CAD build for the part. Positions are in the model's coordinates, mm. Give positions to 0.01 mm unless a question says otherwise; leave off trailing zeros. Loops run counter-clockwise (first coordinate to the right, second up) from the corner with the lowest first, then second, coordinate; pieces in that order, holes last. Notation, with made-up numbers: M 47,89 L 56,89 A14 ccw 56,103 Z; hole C 73.5,36 d3. An arc over 180 degrees is marked long. Answer as CSV lines item,"result".
```python
from build123d import *

# Parameters (mm, degrees)
SKETCH_1_R       = 4.175
EXTRUDE_1_DEPTH  = 5
FILLET_1_DEPTH   = 5
FILLET_1_2_DEPTH = 5


with BuildPart() as part:
    # ｽｹｯﾁ1 → ﾎﾞｽ - 押し出し1 (new body)
    # profile 1 of 4: a face of its own
    with BuildSketch(Plane(origin=(0, 0, 0), x_dir=(1, 0, 0), z_dir=(0, 1, 0))):
        Polygon((21.537147831, 13.436802865), (14.676517829, 20.712224225), (-21.537147831, -13.436802865), (-14.676517829, -20.712224225), align=None)
        with Locations(Location((-12.65026681, -11.929041043, 0), (0, 0, 270))):
            Circle(SKETCH_1_R, mode=Mode.SUBTRACT)
        with Locations(Location((5.538286591, 5.222533963, 0), (0, 0, 270))):
            Circle(SKETCH_1_R, mode=Mode.SUBTRACT)
    # profile 2 of 4: a face of its own
    with BuildSketch(Plane(origin=(0, 0, 0), x_dir=(1, 0, 0), z_dir=(0, 1, 0))):
        Polygon((21.537147831, 13.436802865), (-14.676517829, -20.712224225), (-21.537147831, -13.436802865), (14.676517829, 20.712224225), align=None)
        with Locations(Location((5.538286591, 5.222533963, 0), (0, 0, 270))):
            Circle(SKETCH_1_R, mode=Mode.SUBTRACT)
        with Locations(Location((-12.65026681, -11.929041043, 0), (0, 0, 270))):
            Circle(SKETCH_1_R, mode=Mode.SUBTRACT)
    # profile 3 of 4: a face of its own
    with BuildSketch(Plane(origin=(0, 0, 0), x_dir=(1, 0, 0), z_dir=(0, 1, 0))):
        with BuildLine():
            ThreePointArc((19.221377033, 19.536564594), (16.900027476, 19.935279891), (14.676517829, 20.712224225))
            Line((14.676517829, 20.712224225), (21.537147831, 13.436802865))
            ThreePointArc((21.537147831, 13.436802865), (22.425633577, 14.316933157), (23.303261531, 15.207890747))
            Line((23.303261531, 15.207890747), (19.221377033, 19.536564594))
        make_face()
    # profile 4 of 4: a face of its own
    with BuildSketch(Plane(origin=(0, 0, 0), x_dir=(1, 0, 0), z_dir=(0, 1, 0))):
        with BuildLine():
            ThreePointArc((10.415298606, 43.723687992), (6.493592725, 31.097199803), (14.676517829, 20.712224225))
            ThreePointArc((14.676517829, 20.712224225), (16.900027476, 19.935279891), (19.221377033, 19.536564594))
            Line((19.221377033, 19.536564594), (16.881068514, 22.018367371))
            ThreePointArc((16.881068514, 22.018367371), (8.617568994, 30.735491067), (11.829512169, 42.309474429))
            Line((11.829512169, 42.309474429), (10.415298606, 43.723687992))
        make_face()
    extrude(amount=EXTRUDE_1_DEPTH)

    # ﾌｨﾚｯﾄ1: read off the stored shape, not the designer's step
    # ﾌｨﾚｯﾄ1 outline → ﾌｨﾚｯﾄ1 (cut)
    with BuildSketch(Plane(origin=(0, 0, 0), x_dir=(1, 0, 0), z_dir=(0, 1, 0))):
        with BuildLine():
            Line((23.303261531, 15.207890747), (16.881068514, 22.018367371))
            ThreePointArc((16.881068514, 22.018367371), (19.214955148, 15.00333268), (16.092088027, 8.302180578))
            Line((16.092088027, 8.302180578), (21.537147831, 13.436802865))
            ThreePointArc((21.537147831, 13.436802865), (22.425633577, 14.316933157), (23.303261531, 15.207890747))
        make_face()
    extrude(amount=FILLET_1_DEPTH, mode=Mode.SUBTRACT)

    # Fillet 1 2 outline → Fillet 1 2 (add)
    with BuildSketch(Plane(origin=(0, 0, 0), x_dir=(1, 0, 0), z_dir=(0, 1, 0))):
        with BuildLine():
            ThreePointArc((14.676517829, 20.712224225), (11.188521166, 22.924061141), (8.484552975, 26.046063588))
            ThreePointArc((8.484552975, 26.046063588), (9.977695299, 19.436676513), (6.914435143, 13.39267877))
            Line((6.914435143, 13.39267877), (14.676517829, 20.712224225))
        make_face()
    extrude(amount=FILLET_1_2_DEPTH)


solid = part.part
```
Q1. Cut at A-A (x = -15.5). Write the cut outline in (y, z).
Solution:
outline,"M 0,7.74 L 5,7.74 L 5,8.88 L 0,8.88 Z; M 0,14.98 L 5,14.98 L 5,19.84 L 0,19.84 Z"
Q2. Pin check, flat tip, straight feed: P1, Ø8, axis at x = -4.5, z = -9.5, coming from the +Y side (1 decimal). Stop position of the tip, or through.
Solution:
P1,"passes through"
Q3. Cut at D-D (x = -7). Write the cut outline in (y, z), and give its area (3 significant figures).
Solution:
outline,"M 0,-0.27 L 5,-0.27 L 5,13.47 L 0,13.47 Z"
area,"68.7 mm²"
Q4. Mould opens along Z. For faces 1 (the cylindrical face through (19.22, 2.46, -15.11)), 2 (the cylindrical face through (8.66, 2.46, -30.57)), 3 (the flat face through (0, 5, -4)) say: released by +Z, released by -Z, zero draft, split by the parting line, or undercut.
Solution:
face 1,"split by the parting line"
face 2,"undercut"
face 3,"zero draft"
Q5. Cut at C-C (z = -3). Write the cut outline in (x, y), and give its area (3 significant figures).
Solution:
outline,"M -4.11,0 L 2,0 L 2,5 L -4.11,5 Z; M 9.07,0 L 10.47,0 L 10.47,5 L 9.07,5 Z"
area,"37.5 mm²"
Q6. Wall check: line 1 (Z direction, x = -10, y = 4.1); line 2 (Z direction, x = -10.5, y = 2.5); line 3 (Z direction, x = 13, y = 1.5). Give the ranges that are in metal, low to high. Write a range as [from, to].
Solution:
line 1,"z = [2.56, 8.7], [15.15, 16.3]"
line 2,"z = [3.03, 8.35], [15.51, 16.77]"
line 3,"z = [-24.03, -5.39]"
Q7. Cut at B-B (y = 1). Write the cut outline in (x, z) (3 decimals).
Solution:
outline,"M -21.537,13.437 L 6.914,-13.393 A10 cw 8.485,-26.046 A14.2 ccw 10.415,-43.724 L 11.83,-42.309 A12.2 cw 16.881,-22.018 A10 ccw 16.092,-8.302 L -14.677,20.712 Z; hole C -12.65,11.929 d8.35; hole C 5.538,-5.223 d8.35"
